```python
from build123d import *

# Parameters (mm, degrees)
EXTRUDE_1_DEPTH     = 80
SKETCH_2_R          = 1.45
CUT_EXTRUDE_1_DEPTH = 80
FILLET_1_R          = 6
CUT_EXTRUDE_2_DEPTH = 10


with BuildPart() as part:
    # 草图1 → 凸台-拉伸1 (new body)
    with BuildSketch(Plane.XY):
        with BuildLine():
            Line((-37, 0), (-27.5, 0))
            Line((-27.5, 0), (-27.5, 6.6))
            ThreePointArc((-27.5, 6.6), (-24.746803743, 13.246803743), (-18.1, 16))
            Line((-18.1, 16), (18.1, 16))
            ThreePointArc((18.1, 16), (24.746803743, 13.246803743), (27.5, 6.6))
            Line((27.5, 6.6), (27.5, 0))
            Line((27.5, 0), (37, 0))
            Line((37, 0), (37, 2))
            Line((37, 2), (29.5, 2))
            Line((29.5, 2), (29.5, 6.6))
            ThreePointArc((29.5, 6.6), (26.161017306, 14.661017306), (18.1, 18))
            Line((18.1, 18), (-18.1, 18))
            ThreePointArc((-18.1, 18), (-26.161017306, 14.661017306), (-29.5, 6.6))
            Line((-29.5, 6.6), (-29.5, 2))
            Line((-29.5, 2), (-37, 2))
            Line((-37, 2), (-37, 0))
        make_face()
    extrude(amount=EXTRUDE_1_DEPTH)

    # 草图2 → 切除-拉伸1 (cut)
    with BuildSketch(Plane(origin=(0, 2, 0), x_dir=(1, 0, 0), z_dir=(0, 1, 0))):
        with Locations(Location((-33, -19, 0), (0, 0, 180))):
            Circle(SKETCH_2_R)
        with Locations(Location((-33, -61, 0), (0, 0, 270))):
            Circle(SKETCH_2_R)
        with Locations(Location((33, -61, 0), (0, 0, 180))):
            Circle(SKETCH_2_R)
        with Locations(Location((33, -19, 0), (0, 0, 180))):
            Circle(SKETCH_2_R)
    extrude(amount=-CUT_EXTRUDE_1_DEPTH, mode=Mode.SUBTRACT)

    # 圆角1
    fillet_1_edges = [part.edges().sort_by_distance(p)[0] for p in [
        (37, 1, 0),
        (-37, 1, 0),
        (37, 1, 80),
        (-37, 1, 80),
    ]]
    fillet(fillet_1_edges, radius=FILLET_1_R)

    # 草图3 → 切除-拉伸2 (cut)
    with BuildSketch(Plane(origin=(0, 18, 0), x_dir=(1, 0, 0), z_dir=(0, 1, 0))):
        Polygon((0.684609691, -72.718226784), (10.684609691, -72.718226784), (15.1, -70.169), (15.1, -64.395497308), align=None)
        Polygon((-15.1, -72.718226784), (-10.1, -72.718226784), (15.1, -58.169), (15.1, -52.395497308), (-15.1, -69.831475438), align=None)
        Polygon((-15.1, -57.831475438), (-15.1, -63.60497813), (15.1, -46.169), (15.1, -40.395497308), align=None)
        Polygon((-15.1, -45.831475438), (-15.1, -51.60497813), (15.1, -34.169), (15.1, -28.395497308), align=None)
        Polygon((-15.1, -33.831475438), (-15.1, -39.60497813), (15.1, -22.169), (15.1, -16.395497308), align=None)
        Polygon((10.1, -7.282248654), (15.1, -7.282248654), (15.1, -10.169), (-15.1, -27.60497813), (-15.1, -21.831475438), align=None)
        Polygon((-15.1, -9.831475438), (-15.1, -15.60497813), (-0.684609691, -7.282248654), (-10.684609691, -7.282248654), align=None)
    extrude(amount=-CUT_EXTRUDE_2_DEPTH, mode=Mode.SUBTRACT)


solid = part.part
```
Design review of the part built by this model. Coordinates are the model's own, in mm. A direction names the side the tool comes from. Coordinates: 2 decimals unless noted, no trailing zeros. Order: outer loops, then holes, each group sorted by start corner. A loop starts at its lowest first (then second) coordinate and runs counter-clockwise, first axis right, second up. Notation, with made-up numbers: (80, 83.25) -> (85, 83.25) arc R8 ccw to (85, 98.25) -> close; hole circle Ø6 at (42.5, -35). An arc over 180 degrees is marked (long way). One line per item, written item: value. Start each with the question number.
Q1. Take a section at A-A, the plane y = 5.25. State the section outline as (x, z) points.
Q2. For probe 1 along X at (y, z) = (5, 18); probe 2 along Z at (x, y) = (33, 1.45); probe 3 along X at (y, z) = (1, 44.5), list the stretches that pass through material, from the lowest coordinate up.
Q3. Take a section at C-C, the plane x = -3.5. State the section outline as (y, z) points, then the cut area to 3 significant figures.
Q4. Take a section at D-D, the plane x = 33. State the section outline as (y, z) points.
Q5. Take a section at B-B, the plane z = 61. Give the number of separate pieces and of enclosed holes in the cut face, then the cut area to 3 significant figures.
Q6. Tool access review of faces 4 (the flat face through (-37, 1, 40)), 5 (the cylindrical face through (24.67, 13.32, 39.44)), 6 (the flat face through (-33, 2, 39)), 7 (the flat face through (15.1, 17, 43)): name each direction out of +Z, -Z, +X, -X, +Y, -Y from which nothing blocks a thin tool from reaching the whole face with its end or side.
Q7. Insertion check: pin 1 Ø6 at (x, z) = (-33.5, 42.5) entering from +Y; pin 2 Ø3 at (y, z) = (8.5, 27) entering from -X; pin 3 Ø2 at (y, z) = (17.5, 72) entering from +X. Each pin has a flat end and moves straight along its axis. Give the tip position at first contact, or say it passes through.
Q8. Mouldability with a two-part tool opening along Z and no side actions: class faces 1 (the flat face through (-2.4, 16.4, 80)), 2 (the cylindrical face through (26.25, 14.57, 39.44)), 3 (the flat face through (15.1, 17, 67)) as pulls with the +Z half, pulls with the -Z half, needs draft (parallel to the pull), parting line crosses it, or undercut.
Values follow:
1. outline: (-29.5, 0) -> (-27.5, 0) -> (-27.5, 80) -> (-29.5, 80) -> close; (27.5, 0) -> (29.5, 0) -> (29.5, 80) -> (27.5, 80) -> close
2. probe 1: x = -29.5 to -27.5, 27.5 to 29.5
2. probe 2: z = 0.34 to 17.55, 20.45 to 59.55, 62.45 to 79.66
2. probe 3: x = -37 to -27.5, 27.5 to 37
3. outline: (16, 0) -> (18, 0) -> (18, 7.28) -> (16, 7.28) -> close; (16, 8.91) -> (18, 8.91) -> (18, 15.13) -> (16, 15.13) -> close; (16, 20.91) -> (18, 20.91) -> (18, 27.13) -> (16, 27.13) -> close; (16, 32.91) -> (18, 32.91) -> (18, 39.13) -> (16, 39.13) -> close; (16, 44.91) -> (18, 44.91) -> (18, 51.13) -> (16, 51.13) -> close; (16, 56.91) -> (18, 56.91) -> (18, 63.13) -> (16, 63.13) -> close; (16, 68.91) -> (18, 68.91) -> (18, 80) -> (16, 80) -> close
3. area: 99.0 mm2
4. outline: (0, 0.34) -> (2, 0.34) -> (2, 17.55) -> (0, 17.55) -> close; (0, 20.45) -> (2, 20.45) -> (2, 59.55) -> (0, 59.55) -> close; (0, 62.45) -> (2, 62.45) -> (2, 79.66) -> (0, 79.66) -> close
5. separate pieces: 5
5. enclosed holes: 0
5. area: 154 mm2
6. face 4: +Z, -Z, -X, +Y, -Y
6. face 5: +Z, -Z, -Y
6. face 6: +Z, -Z, -X, +Y
6. face 7: +Y, -Y
7. pin 1: stops at y = 2
7. pin 2: stops at x = -29.49
7. pin 3: stops at x = 23.75
8. face 1: pulls with the +Z half
8. face 2: needs draft
8. face 3: undercut
